CAD build for the part. Positions are in the model's coordinates, mm. A direction names the side the tool comes from. Coordinates: 2 decimals unless noted, no trailing zeros. Write each loop counter-clockwise with the first axis right and the second up, starting at its lowest first coordinate (ties: lowest second). Pieces come first, ordered by that corner, then holes. Notation, with made-up numbers: (42.25, -12.5) -> (70.25, -12.5) arc R20 ccw to (70.25, 23.5) -> close; hole circle Ø7 at (15, 41). An arc over 180 degrees is marked (long way). Answer as CSV lines item,"result".
Autodesk Inventor part; units mm, degrees
ref_plane "Work Plane1" through (0, 120, 0) normal (0, 1, 0) x (1, 0, 0)
ref_plane "YZ Plane" through (0, 0, 0) normal (1, 0, 0) x (0, 1, 0)
ref_plane "XZ Plane" through (0, 0, 0) normal (0, 1, 0) x (-1, 0, 0)
sketch "Sketch1" plane through (0, 0, 0) normal (0, 1, 0) x (-1, 0, 0)
  line L0 (1, 65) -> (-1, 65)
  line L1 (-1, 65) -> (-1, -65)
  line L2 (-1, -65) -> (1, -65)
  line L3 (1, -65) -> (1, 65)
  line L4 (1, 65) -> (-1, -65) construction
  point P0 (0, 0)
  point P1 (0, 0)
  dimension "d0" = 130
  dimension "d1" = 2
extrude "Extrusion1" add sketch "Sketch1" along normal blind 128
ref_plane "Work Plane1" through (0, 120, 0) normal (0, 1, 0) x (1, 0, 0)
sketch "Sketch2" plane through (0, 120, 0) normal (0, 1, 0) x (1, 0, 0)
  line L0 (-1, -65) -> (1, -65)
  line L1 (1, 65) -> (-1, 65)
  line L2 (-1, -65) -> (-7, -65)
  line L3 (-7, -65) -> (-7, 65)
  line L4 (-7, 65) -> (-1, 65)
  line L5 (-1, 65) -> (-1, -65)
  point P0 (0, 0)
  dimension "d5" = 6
extrude "Extrusion2" add sketch "Sketch2" along normal blind 1
sketch "Sketch3" plane through (-1, 0, -65) normal (-1, 0, 0) x (0, 0, 1)
  line L0 (0, 5) -> (130, 5)
  line L1 (130, 5) -> (130, 5.5)
  line L2 (130, 5.5) -> (0, 5.5)
  line L3 (0, 5.5) -> (0, 5)
  line L4 (0, 0) -> (0, 120)
  line L5 (130, 0) -> (130, 120)
  line L6 (0, 0) -> (130, 0)
  line L7 (0, 15) -> (130, 15)
  line L8 (130, 15) -> (130, 15.5)
  line L9 (130, 15.5) -> (0, 15.5)
  line L10 (0, 15.5) -> (0, 15)
  line L11 (0, 25) -> (130, 25)
  line L12 (130, 25) -> (130, 25.5)
  line L13 (130, 25.5) -> (0, 25.5)
  line L14 (0, 25.5) -> (0, 25)
  line L15 (0, 35) -> (130, 35)
  line L16 (130, 35) -> (130, 35.5)
  line L17 (130, 35.5) -> (0, 35.5)
  line L18 (0, 35.5) -> (0, 35)
  line L19 (0, 45) -> (130, 45)
  line L20 (130, 45) -> (130, 45.5)
  line L21 (130, 45.5) -> (0, 45.5)
  line L22 (0, 45.5) -> (0, 45)
  line L23 (0, 55) -> (130, 55)
  line L24 (130, 55) -> (130, 55.5)
  line L25 (130, 55.5) -> (0, 55.5)
  line L26 (0, 55.5) -> (0, 55)
  line L27 (0, 65) -> (130, 65)
  line L28 (130, 65) -> (130, 65.5)
  line L29 (130, 65.5) -> (0, 65.5)
  line L30 (0, 65.5) -> (0, 65)
  line L31 (0, 75) -> (130, 75)
  line L32 (130, 75) -> (130, 75.5)
  line L33 (130, 75.5) -> (0, 75.5)
  line L34 (0, 75.5) -> (0, 75)
  line L35 (0, 85) -> (130, 85)
  line L36 (130, 85) -> (130, 85.5)
  line L37 (130, 85.5) -> (0, 85.5)
  line L38 (0, 85.5) -> (0, 85)
  line L39 (0, 95) -> (130, 95)
  line L40 (130, 95) -> (130, 95.5)
  line L41 (130, 95.5) -> (0, 95.5)
  line L42 (0, 95.5) -> (0, 95)
  line L43 (0, 105) -> (130, 105)
  line L44 (130, 105) -> (130, 105.5)
  line L45 (130, 105.5) -> (0, 105.5)
  line L46 (0, 105.5) -> (0, 105)
  line L47 (0, 115) -> (130, 115)
  line L48 (130, 115) -> (130, 115.5)
  line L49 (130, 115.5) -> (0, 115.5)
  line L50 (0, 115.5) -> (0, 115)
  point P0 (65, 0)
  dimension "d8" = 0.5
  dimension "d9" = 5
  dimension "d12" = 10
extrude "Extrusion3" add sketch "Sketch3" along normal blind 0.5 contours L3 L2 L1 L0 | L4 L9 L5 L7 | L4 L13 L5 L11 | L4 L17 L5 L15 | L4 L21 L5 L19 | L4 L25 L5 L23 | L4 L29 L5 L27 | L4 L33 L5 L31 | L4 L37 L5 L35 | L4 L41 L5 L39 | L4 L45 L5 L43 | L4 L49 L5 L47
properties part number "Platina forntal interna" material "Stainless Steel"
Item 1: Wall check: line 1 (X direction, y = 118.5, z = -24.5); line 2 (Y direction, x = -4, z = -60). Give the ranges that are in metal, low to high. Write a range as from..to.
Answer below:
line 1,"x = -1..1"
line 2,"y = 120..121"
Item 2: 3-axis set-ups, long thin cutter, end or side, ignore diameter. For faces 4 (the flat face through (-1, 2, -1)), 5 (the flat face through (-1, 124, -1)), 6 (the flat face through (1, 63, 1)), 7 (the flat face through (-1, 10, -1)): which of +Z, -Z, +X, -X, +Y, -Y reach the whole face in a straight line?
Answer below:
face 4,"+Z, -Z, -X, -Y"
face 5,"+Z, -Z, -X, +Y"
face 6,"+Z, -Z, +X, +Y, -Y"
face 7,"+Z, -Z, -X"
Item 3: Saw through at A-A on x = -3. Give the cut face in (y, z), and give its area (3 significant figures).
Answer below:
outline,"(120, -65) -> (121, -65) -> (121, 65) -> (120, 65) -> close"
area,"130 mm2"
Item 4: Flat gauge pins, fed straight in: pin 1 (1.8 mm diameter, centred on x = -5, z = -28.5, fed in from -Y); pin 2 (5 mm diameter, centred on y = 10, z = -12, fed in from -X); pin 3 (0.6 mm diameter, centred on y = 115.5, z = 23.5, fed in from -X). Where does each tip first touch, or does it go through?
Answer below:
pin 1,"stops at y = 120"
pin 2,"stops at x = -1"
pin 3,"stops at x = -1.5"
Item 5: Saw through at B-B on y = 61. Give the cut face in (x, z).
Answer below:
outline,"(-1, -65) -> (1, -65) -> (1, 65) -> (-1, 65) -> close"
Item 6: Two-plate mould, pull along Y, no slides. Class faces 1 (the flat face through (-1, 70, -1)), 2 (the flat face through (-4, 121, -1)), 3 (the flat face through (0, 73, 65)): pulls with the +Y half, pulls with the -Y half, needs draft (parallel to the pull), parting line crosses it, or undercut.
Answer below:
face 1,"undercut"
face 2,"pulls with the +Y half"
face 3,"needs draft"
